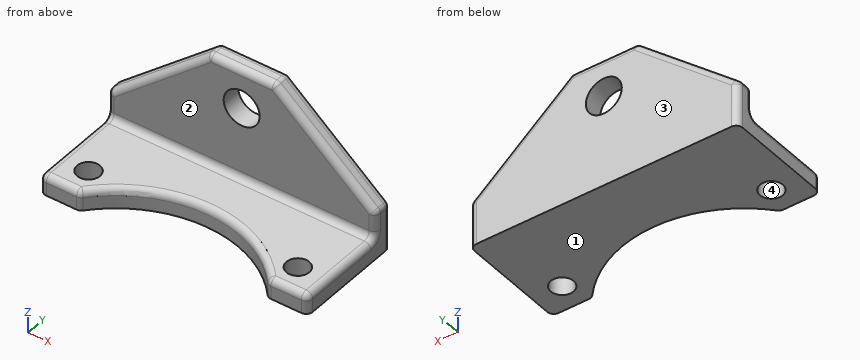
from build123d import *

# Parameters (mm, degrees)
SKETCH1_R           = 1.75
BOSS_EXTRUDE1_DEPTH = 3
SKETCH2_R           = 2.75
BOSS_EXTRUDE2_DEPTH = 3
FILLET1_R           = 1


with BuildPart() as part:
    # Sketch1 → Boss-Extrude1 (new body)
    with BuildSketch(Plane.XY):
        with BuildLine():
            Line((-20.5, 7), (-20.5, -7))
            Line((-20.5, -7), (-14.407029534, -7))
            ThreePointArc((-14.407029534, -7), (0, -0.25), (14.407029534, -7))
            Line((14.407029534, -7), (20.5, -7))
            Line((20.5, -7), (20.5, 7))
            Line((20.5, 7), (-20.5, 7))
        make_face()
        with Locations((-16, -3)):
            Circle(SKETCH1_R, mode=Mode.SUBTRACT)
        with Locations(Location((16, -3, 0), (0, 0, 180))):
            Circle(SKETCH1_R, mode=Mode.SUBTRACT)
    extrude(amount=BOSS_EXTRUDE1_DEPTH)

    # Sketch2 → Boss-Extrude2 (add)
    with BuildSketch(Plane(origin=(0, 7, 0), x_dir=(1, 0, 0), z_dir=(0, 1, 0))):
        Polygon((-20.5, 0), (20.5, 0), (20.5, -7), (5.007203296, -20), (-5.007203296, -20), (-20.5, -7), align=None)
        with Locations(Location((0, -14, 0), (0, 0, 270))):
            Circle(SKETCH2_R, mode=Mode.SUBTRACT)
    extrude(amount=BOSS_EXTRUDE2_DEPTH)

    # Fillet1
    fillet1_edges = [part.edges().sort_by_distance(p)[0] for p in [
        (20.5, 0, 3),
        (-14.407029534, -7, 1.5),
        (-20.5, -7, 1.5),
        (20.5, -7, 1.5),
        (14.407029534, -7, 1.5),
        (0, 7, 3),
        (-20.5, 0, 3),
        (-17.453514767, -7, 3),
        (-12.753601648, 10, 13.5),
        (0, 10, 20),
        (12.753601648, 10, 13.5),
        (20.5, 10, 3.5),
        (-20.5, 10, 3.5),
        (-12.753601648, 7, 13.5),
        (-20.5, 8.5, 7),
        (0, 7, 20),
        (-5.007203296, 8.5, 20),
        (12.753601648, 7, 13.5),
        (5.007203296, 8.5, 20),
        (20.5, 7, 5),
        (20.5, 8.5, 7),
        (-20.5, 7, 5),
        (0, -0.25, 3),
        (17.453514767, -7, 3),
    ]]
    fillet(fillet1_edges, radius=FILLET1_R)


solid = part.part
Design review of the part built by this model. Coordinates are the model's own, in mm. Face numbers are marked on the shaded views. A direction names the side the tool comes from. Round coordinates to 2 decimals unless told otherwise and drop trailing zeros. Loops run counter-clockwise (first coordinate to the right, second up) from the corner with the lowest first, then second, coordinate; pieces in that order, holes last. Notation, with made-up numbers: M 83.5,15 L 139.5,15 A11 ccw 139.5,28 Z; hole C 30.25,8 d6. An arc over 180 degrees is marked long. Answer as a JSON object with one key per item and string values.
Item 1: We need section B-B on y = 4.25. Give the boundary of the cut face in (x, z), and give its area (3 significant figures).
Answer sheet:
{"outline": "M -20.5,0 L 20.5,0 L 20.5,2 A1 ccw 19.5,3 L -19.5,3 A1 ccw -20.5,2 Z", "area": "123 mm^2"}
Item 2: Clearance check with flat-ended pins moving along their axes: P1, Ø7.5, axis at x = -6, z = 8, coming from the -Y side; P2, Ø9.5, axis at x = 0, y = -2, coming from the +Z side. State where each tip first meets the part, or that it passes through.
Answer sheet:
{"P1": "stops at y = 7", "P2": "stops at z = 3"}
Item 3: Wall thickness on L1, parallel to Y at x = 4.5, z = 10.25; L2, parallel to Z at x = -9, y = 2.5; L3, parallel to X at y = -2.75, z = 2: over which ranges is each line inside the solid? List them lowest first. Write a range as from..to.
Answer sheet:
{"L1": "y = 7..10", "L2": "z = 0..3", "L3": "x = -20.5..-17.73, -14.27..-9.35, 9.35..14.27, 17.73..20.5"}
Item 4: Machinability: for the marked faces 1 and 2, which of the approach directions +Z, -Z, +X, -X, +Y, -Y give a long, thin tool a straight path to every point of the face, cutting with its end or side? Answer none if there is none.
Answer sheet:
{"face 1": "-Z, +X, -X, +Y, -Y", "face 2": "+Z, +X, -X, -Y"}
Item 5: The part is to be moulded in two halves that separate along X. For the marked faces 3 and 4, say which applies: pulls with the +X half, pulls with the -X half, needs draft (parallel to the pull), parting line crosses it, or undercut.
Answer sheet:
{"face 3": "needs draft", "face 4": "undercut"}
Item 6: We need section A-A on x = 0. Give the boundary of the cut face in (y, z).
Answer sheet:
{"outline": "M -0.25,0 L 10,0 L 10,11.25 L 7,11.25 L 7,4 A1 cw 6,3 L 0.75,3 A1 ccw -0.25,2 Z; M 7,16.75 L 10,16.75 L 10,19 A1 ccw 9,20 L 8,20 A1 ccw 7,19 Z"}
Item 7: We need section C-C on y = -3. State how many separate pieces and enclosed holes the cut face has, and give its area (3 significant figures).
Answer sheet:
{"separate pieces": "4", "enclosed holes": "0", "area": "42.1 mm^2"}
